Here's how the part is built. I have some questions about the finished solid (model axes, mm). A direction names the side the tool comes from. Round coordinates to 2 decimals unless told otherwise and drop trailing zeros. Write each loop counter-clockwise with the first axis right and the second up, starting at its lowest first coordinate (ties: lowest second). Pieces come first, ordered by that corner, then holes. Notation, with made-up numbers: M -10,4.5 L 7,4.5 A23 cw 7,13.5 Z; hole C 56.25,51 d6. An arc over 180 degrees is marked long. Use a Markdown table: item, result. Add a question column.
```python
from build123d import *

# Parameters (mm, degrees)
SKETCH1_R               = 12.7
SKETCH1_R_2             = 10.16
BOSS_EXTRUDE1_DEPTH     = 38.1
BOSS_EXTRUDE2_START     = -5.08
SKETCH2_R               = 12.7
BOSS_EXTRUDE2_DEPTH     = 5.08
CUT_EXTRUDE1_START      = -2.54
CUT_EXTRUDE1_DEPTH      = 2.54
FILLET1_R               = 10
CUT_EXTRUDE2_DEPTH      = 48.519048812
CUT_EXTRUDE2_DEPTH_BACK = 48.519048812
SKETCH5_R               = 1.5


with BuildPart() as part:
    # Sketch1 → Boss-Extrude1 (new body)
    with BuildSketch(Plane(origin=(0, 0, 0), x_dir=(1, 0, 0), z_dir=(0, 1, 0))):
        with Locations(Location((0, 0, 0), (0, 0, 90))):
            Circle(SKETCH1_R)
        with Locations(Location((0, 0, 0), (0, 0, 90))):
            Circle(SKETCH1_R_2, mode=Mode.SUBTRACT)
    extrude(amount=BOSS_EXTRUDE1_DEPTH)

    # Sketch2 → Boss-Extrude2 (add)
    with BuildSketch(Plane(origin=(0, 38.1, 0), x_dir=(1, 0, 0), z_dir=(0, 1, 0)).offset(BOSS_EXTRUDE2_START)):
        with Locations(Location((0, 0, 0), (0, 0, 90))):
            Circle(SKETCH2_R)
    extrude(amount=BOSS_EXTRUDE2_DEPTH)

    # Sketch3 → Cut-Extrude1 (cut)
    with BuildSketch(Plane(origin=(0, 38.1, 0), x_dir=(1, 0, 0), z_dir=(0, 1, 0)).offset(CUT_EXTRUDE1_START)):
        with BuildLine():
            Line((0, 3.5), (-12.418726065, 2.65805247))
            ThreePointArc((-12.418726065, 2.65805247), (-12.7, 0), (-12.418726065, -2.65805247))
            Line((-12.418726065, -2.65805247), (0, -3.5))
            Line((0, -3.5), (12.418726065, -2.65805247))
            ThreePointArc((12.418726065, -2.65805247), (12.7, 0), (12.418726065, 2.65805247))
            Line((12.418726065, 2.65805247), (0, 3.5))
        make_face()
    extrude(amount=CUT_EXTRUDE1_DEPTH, mode=Mode.SUBTRACT)

    # Fillet1
    fillet1_edges = [part.edges().sort_by_distance(p)[0] for p in [
        (0, 36.83, 3.5),
        (0, 36.83, -3.5),
    ]]
    fillet(fillet1_edges, radius=FILLET1_R)

    # Sketch5 → Cut-Extrude2 (cut, two sides: drawn at the far end of the back side and taken through both)
    with BuildSketch(Plane.XY.offset(-12.7).offset(-CUT_EXTRUDE2_DEPTH_BACK)):
        with Locations(Location((0, 28.1, 0), (0, 0, 270.000000018))):
            Circle(SKETCH5_R)
        with Locations(Location((0, 10, 0), (0, 0, 270.000000018))):
            Circle(SKETCH5_R)
    extrude(amount=CUT_EXTRUDE2_DEPTH + CUT_EXTRUDE2_DEPTH_BACK, mode=Mode.SUBTRACT)


solid = part.part
```
Item 1: Imagine slicing it at C-C on z = 8.5. List the corners of the cut face in (x, y) for me, plus the area to 3 significant figures.
Item 2: On a 3-axis mill with a long thin cutter (end or side, diameter ignored), from which of +Z, -Z, +X, -X, +Y, -Y can I reach the whole of each face in a straight line? I mean faces 1 (the face through (-6.63, 36.81, 3.05)), 2 (the face through (0.45, 26.67, -11.39)), 3 (the face through (0, 33.02, 0)). Say none if no direction works.
Item 3: For pin 1 Ø8 at (y, z) = (26.5, -7.5) entering from +X; pin 2 Ø4 at (x, y) = (-7.5, 5.5) entering from -Z; pin 3 Ø5 at (y, z) = (30, -9.5) entering from +X, each with a flat end and sliding along its axis, tell me the tip position at first contact or that it passes through.
Item 4: Imagine slicing it at A-A on x = 0. List the corners of the cut face in (y, z) for me.
Item 5: If we mould it in two halves opening along X, with no side actions, what happens to faces 4 (the face through (4.864, 18.783, -11.732)), 5 (the face through (0.45, 8.57, 11.36)), 6 (the face through (-9, 0, 6))? For each: +X half, -X half, draft (parallel to the pull), parting line (faces both ways), or undercut.
Item 6: Imagine slicing it at D-D on y = 20.5. List the corners of the cut face in (x, z) for me.
Item 7: Imagine slicing it at B-B on y = 28.1. List the corners of the cut face in (x, z) for me.
Item 8: I need wall thicknesses on probe 1 along X at (y, z) = (20, 0); probe 2 along Y at (x, z) = (-8.5, -4.25); probe 3 along X at (y, z) = (7, 8.75). Which ranges of each line are inside material? Lowest first, please. Write a range as from..to.
The answers:
| question | item | result |
|---|---|---|
| 1 | outline | M -9.44,0 L -5.57,0 L -5.57,33.02 L 5.57,33.02 L 5.57,0 L 9.44,0 L 9.44,38.1 L -9.44,38.1 Z |
| 1 | area | 351 mm² |
| 2 | face 1 | +Y |
| 2 | face 2 | +Z, -Z |
| 2 | face 3 | -Y |
| 3 | pin 1 | x = 12.21 |
| 3 | pin 2 | z = -11.45 |
| 3 | pin 3 | x = 10.6 |
| 4 | outline | M 0,-12.7 L 8.5,-12.7 L 8.5,-10.16 L 0,-10.16 Z; M 0,10.16 L 8.5,10.16 L 8.5,12.7 L 0,12.7 Z; M 11.5,-12.7 L 26.6,-12.7 L 26.6,-10.16 L 11.5,-10.16 Z; M 11.5,10.16 L 26.6,10.16 L 26.6,12.7 L 11.5,12.7 Z; M 29.6,-12.7 L 38.1,-12.7 L 38.1,-3.48 L 35.56,-3.48 L 35.56,3.48 L 38.1,3.48 L 38.1,12.7 L 29.6,12.7 L 29.6,10.16 L 33.02,10.16 L 33.02,-10.16 L 29.6,-10.16 Z |
| 5 | face 4 | parting line |
| 5 | face 5 | undercut |
| 5 | face 6 | draft |
| 6 | outline | C 0,0 d25.4; hole C 0,0 d20.32 |
| 7 | outline | M -1.5,-12.61 L -1.5,-10.05 A10.16 cw -1.5,10.05 L -1.5,12.61 A12.7 ccw Z; M 1.5,-12.61 A12.7 ccw 1.5,12.61 L 1.5,10.05 A10.16 cw 1.5,-10.05 Z |
| 8 | probe 1 | -12.7..-10.16, 10.16..12.7 |
| 8 | probe 2 | 33.02..38.1 |
| 8 | probe 3 | -9.2..-5.16, 5.16..9.2 |
